Geometry check sheet. Reference: drawing and pictorial views, mm from the part's lowest x, y, z. Coordinates: 2 decimals unless noted, no trailing zeros. Loops run counter-clockwise (first coordinate to the right, second up) from the corner with the lowest first, then second, coordinate; pieces in that order, holes last.
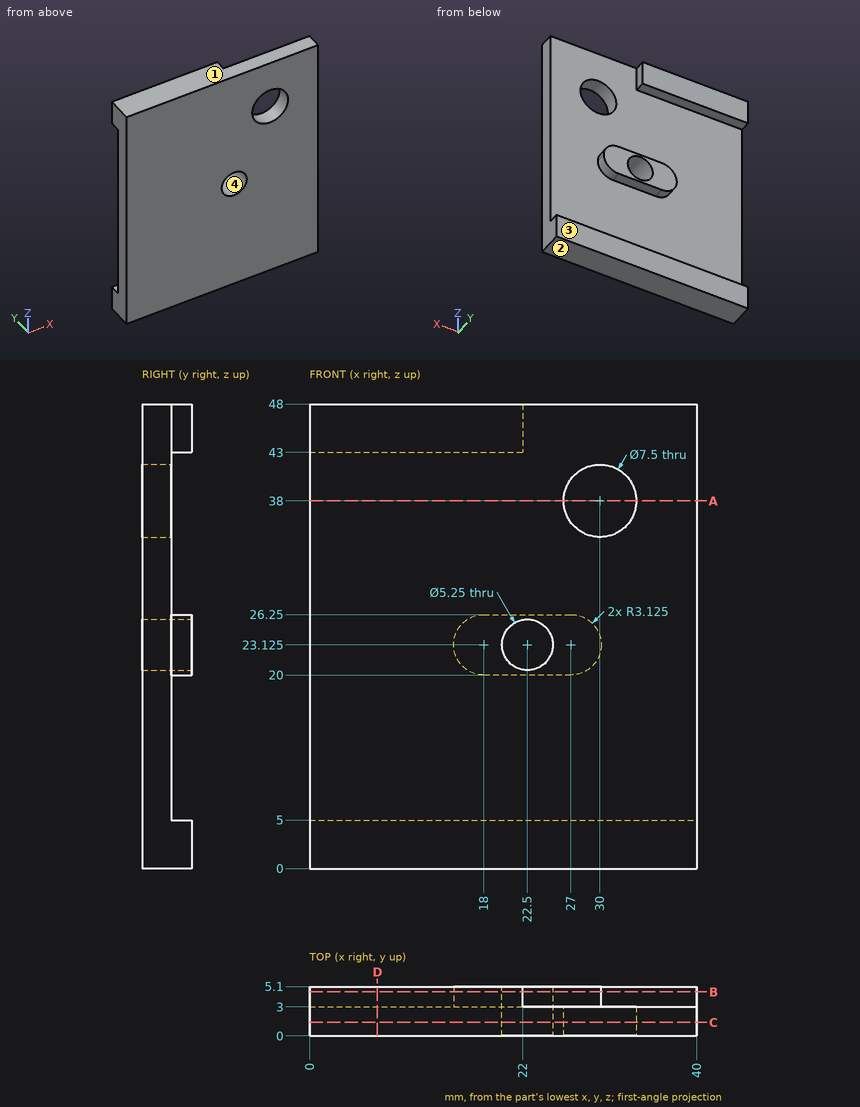
1) Material ranges on probe 1 along Z at (x, y) = (22.5, 1.3); probe 2 along X at (y, z) = (2.3, 38); probe 3 along Z at (x, y) = (30, 1.1), recorded low to high.
Data:
probe 1: z = 0 to 20.5, 25.75 to 48
probe 2: x = 0 to 26.25, 33.75 to 40
probe 3: z = 0 to 34.25, 41.75 to 48
2) Mould release check, pull along Z, two halves, no side actions. Record for the marked faces 1, 2, 3 and 4: +Z half, -Z half, draft (parallel to the pull), parting line (faces both ways), or undercut.
Data:
face 1: +Z half
face 2: -Z half
face 3: draft
face 4: undercut
3) Section check B-B on y = 4.55. Record the cut outline in (x, z) (3 decimals), and give its area (3 significant figures).
Data:
outline: (0, 0) - (40, 0) - (40, 5) - (0, 5) - close; (0, 43) - (22, 43) - (22, 48) - (0, 48) - close; (18, 20) - (27, 20) arc R3.125 ccw to (27, 26.25) - (18, 26.25) arc R3.125 ccw to start; hole circle Ø5.25 at (22.5, 23.125)
area: 375 mm2
4) Section check C-C on y = 1.4. Record the cut outline in (x, z) (3 decimals), and give its area (3 significant figures).
Data:
outline: (0, 0) - (40, 0) - (40, 48) - (0, 48) - close; hole circle Ø5.25 at (22.5, 23.125); hole circle Ø7.5 at (30, 38)
area: 1,850 mm2
5) Section check A-A on z = 38. Record the cut outline in (x, y), and give its area (3 significant figures).
Data:
outline: (0, 0) - (26.25, 0) - (26.25, 3) - (0, 3) - close; (33.75, 0) - (40, 0) - (40, 3) - (33.75, 3) - close
area: 97.5 mm2
6) Depth check by flat-ended pin: pin 1 (4.5 mm diameter, centred on x = 22.5, z = 23.125, fed in from -Y); pin 2 (10 mm diameter, centred on x = 30, z = 38, fed in from +Y). Enter the tip coordinate at first touch or a pass-through.
Data:
pin 1: passes through
pin 2: stops at y = 3
7) Section check D-D on x = 7. Record the cut outline in (y, z).
Data:
outline: (0, 0) - (5.1, 0) - (5.1, 5) - (3, 5) - (3, 43) - (5.1, 43) - (5.1, 48) - (0, 48) - close
